Can you work these out from the drawing? Everything is in mm from the part's minimum corner. A direction names the side the tool comes from. Coordinates: 2 decimals unless noted, no trailing zeros. Write each loop counter-clockwise with the first axis right and the second up, starting at its lowest first coordinate (ties: lowest second). Pieces come first, ordered by that corner, then holes. Notation, with made-up numbers: M 74,27.25 L 125,27.25 A9 cw 125,34.25 Z; hole C -24.5,63 d7. An arc over 180 degrees is marked long. Use one line per item in the form item = value. Start each with the question number.
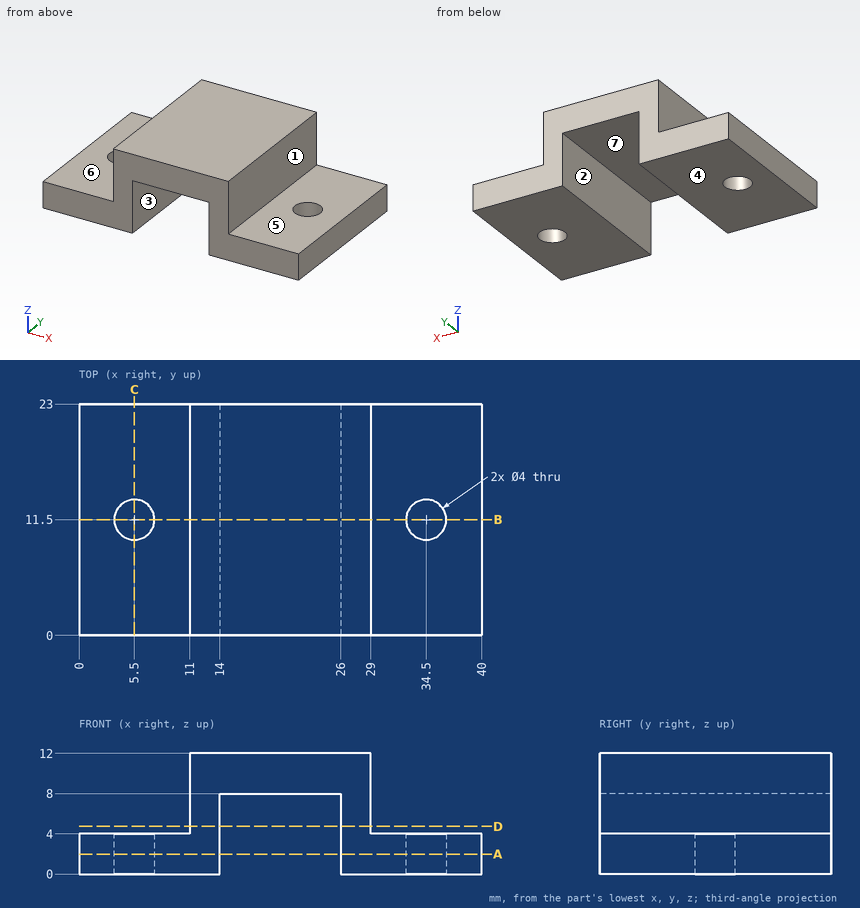
1) Suppose I cut it at D-D on z = 4.75. Please give me the cut outline in (x, y).
2) Which directions (+Z, -Z, +X, -X, +Y, -Y) give clear straight access to the entire face, cutting with the end or side of a thin tool? Please do the marked faces 5, 6 and 7.
3) Suppose I cut it at A-A on z = 2. Please give me the cut outline in (x, y).
4) Please list where these lines run through material, in increasing order: line 1 (X direction, y = 5.25, z = 2.5); line 2 (Y direction, x = 5.5, z = 1.3); line 3 (X direction, y = 12, z = 5).
5) Suppose I cut it at B-B on y = 11.5. Please give me the cut outline in (x, z).
6) Suppose I cut it at C-C on x = 5.5. Please give me the cut outline in (y, z).
7) If we mould it in two halves opening along X, with no side actions, what happens to the marked faces 1, 2, 3 and 4? For each: +X half, -X half, draft (parallel to the pull), parting line (faces both ways), or undercut.
8) Will these pins go through, and if not, where does the flat tip stop? pin 1 Ø3.5 at (x, y) = (37, 6) entering from +Z; pin 2 Ø1.5 at (y, z) = (16.5, 5) entering from +X; pin 3 Ø6 at (x, y) = (18, 13.5) entering from -Z.
Computed values:
q1.outline = M 11,0 L 14,0 L 14,23 L 11,23 Z; M 26,0 L 29,0 L 29,23 L 26,23 Z
q2.face_5 = +Z, +X, +Y, -Y
q2.face_6 = +Z, -X, +Y, -Y
q2.face_7 = -Z, +Y, -Y
q3.outline = M 0,0 L 14,0 L 14,23 L 0,23 Z; M 26,0 L 40,0 L 40,23 L 26,23 Z; hole C 5.5,11.5 d4; hole C 34.5,11.5 d4
q4.line_1 = 0 to 14, 26 to 40
q4.line_2 = 0 to 9.5, 13.5 to 23
q4.line_3 = 11 to 14, 26 to 29
q5.outline = M 0,0 L 3.5,0 L 3.5,4 L 0,4 Z; M 7.5,0 L 14,0 L 14,8 L 26,8 L 26,0 L 32.5,0 L 32.5,4 L 29,4 L 29,12 L 11,12 L 11,4 L 7.5,4 Z; M 36.5,0 L 40,0 L 40,4 L 36.5,4 Z
q6.outline = M 0,0 L 9.5,0 L 9.5,4 L 0,4 Z; M 13.5,0 L 23,0 L 23,4 L 13.5,4 Z
q7.face_1 = +X half
q7.face_2 = undercut
q7.face_3 = undercut
q7.face_4 = draft
q8.pin_1 = 4
q8.pin_2 = 29
q8.pin_3 = 8
